Geometry: final body of the model. Coordinates: model frame, mm. Face numbers are marked on the shaded views. A direction names the side the tool comes from. Give positions to 0.01 mm unless a question says otherwise; leave off trailing zeros. Write each loop counter-clockwise with the first axis right and the second up, starting at its lowest first coordinate (ties: lowest second). Pieces come first, ordered by that corner, then holes.
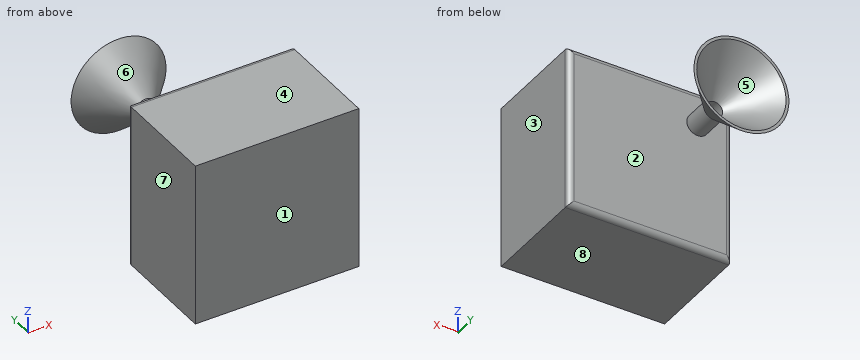
from build123d import *

# Parameters (mm, degrees)
SKETCH1_W           = 300
SKETCH1_H           = 300
BOSS_EXTRUDE1_DEPTH = 200
FILLET1_R           = 10
SKETCH2_R           = 20
SKETCH2_R_2         = 15
BOSS_EXTRUDE2_DEPTH = 50
SKETCH3_R           = 20
BOSS_EXTRUDE3_DEPTH = 80
BOSS_EXTRUDE3_TAPER = -40
SKETCH4_R           = 82
CUT_EXTRUDE1_DEPTH  = 80
CUT_EXTRUDE1_TAPER  = 40


with BuildPart() as part:
    # Sketch1 → Boss-Extrude1 (new body)
    with BuildSketch(Plane(origin=(0, 0, 0), x_dir=(1, 0, 0), z_dir=(0, 1, 0))):
        Rectangle(SKETCH1_W, SKETCH1_H)
    extrude(amount=BOSS_EXTRUDE1_DEPTH)

    # Fillet1
    fillet1_edges = [part.edges().sort_by_distance(p)[0] for p in [
        (-150, 200, 0),
        (0, 200, 150),
        (150, 200, 0),
        (0, 200, -150),
    ]]
    fillet(fillet1_edges, radius=FILLET1_R)

    # Sketch2 → Boss-Extrude2 (add)
    with BuildSketch(Plane(origin=(0, 200, 0), x_dir=(1, 0, 0), z_dir=(0, 1, 0))):
        with Locations((-86.966991411, -86.966991411)):
            Circle(SKETCH2_R)
        with Locations((-86.966991411, -86.966991411)):
            Circle(SKETCH2_R_2, mode=Mode.SUBTRACT)
    extrude(amount=BOSS_EXTRUDE2_DEPTH)

    # Sketch3 → Boss-Extrude3 (add)
    with BuildSketch(Plane(origin=(0, 250, 0), x_dir=(1, 0, 0), z_dir=(0, 1, 0))):
        with Locations((-86.966991411, -86.966991411)):
            Circle(SKETCH3_R)
    extrude(amount=BOSS_EXTRUDE3_DEPTH, taper=BOSS_EXTRUDE3_TAPER)

    # Sketch4 → Cut-Extrude1 (cut)
    with BuildSketch(Plane(origin=(0, 330, 0), x_dir=(1, 0, 0), z_dir=(0, 1, 0))):
        with Locations((-86.966991411, -86.966991411)):
            Circle(SKETCH4_R)
    extrude(amount=-CUT_EXTRUDE1_DEPTH, taper=CUT_EXTRUDE1_TAPER, mode=Mode.SUBTRACT)


solid = part.part
Q1. Access query for the marked faces 4, 5, 6, 7 and 8. Directions: +Z, -Z, +X, -X, +Y, -Y. A direction counts if a zero-diameter tool reaches every point of the face in a straight line with its end or side. Return the directions, or none.
Filled sheet:
face 4: +Z, +X, -X, -Y
face 5: +Y
face 6: none
face 7: +Z, -Z, -X, -Y
face 8: -Z, +X, -X, +Y, -Y
Q2. Pull-direction query (Y, two-part tool) for the marked faces 1, 2 and 3; classes: released by +Y, released by -Y, zero draft, split by the parting line, or undercut.
Filled sheet:
face 1: released by -Y
face 2: undercut
face 3: zero draft
Q3. Ray query, line 1 along X through (y, z) = (146, 146); line 2 along Y through (x, z) = (-39, -2.5). Return the intervals inside material, ascending.
Filled sheet:
line 1: x = -150 to 150
line 2: y = 0 to 200
Q4. Section D-D on y = 159.5. Output: boundary loops of the cut face in (x, z).
Filled sheet:
outline: (-150, -150) - (150, -150) - (150, 150) - (-150, 150) - close
Q5. Section B-B on x = 7. Output: boundary loops of the cut face in (y, z).
Filled sheet:
outline: (0, -150) - (190, -150) arc R10 ccw to (200, -140) - (200, 140) arc R10 ccw to (190, 150) - (0, 150) - close
Q6. Pin query (flat end, axial travel): P1, Ø8, axis at x = -118.5, z = 94.5, coming from the +Y side; P2, Ø24, axis at x = -81.5, z = 89.5, coming from the +Y side; P3, Ø2, axis at x = 96.5, z = 46, coming from the +Y side. Return the tip coordinate at first contact, or that it passes through.
Filled sheet:
P1: stops at y = 275.68
P2: stops at y = 253.76
P3: stops at y = 200
Q7. Section C-C on y = 205. Output: boundary loops of the cut face in (x, z), plus the area to 3 significant figures.
Filled sheet:
outline: circle Ø40 at (-86.97, 86.97); hole circle Ø30 at (-86.97, 86.97)
area: 550 mm2
Q8. Section A-A on z = -127. Output: boundary loops of the cut face in (x, y).
Filled sheet:
outline: (-150, 0) - (150, 0) - (150, 190) arc R10 ccw to (140, 200) - (-140, 200) arc R10 ccw to (-150, 190) - close
